Model file for the job. Use its own axes, mm. A direction names the side the tool comes from. Give positions to 0.01 mm unless a question says otherwise; leave off trailing zeros. Write each loop counter-clockwise with the first axis right and the second up, starting at its lowest first coordinate (ties: lowest second). Pieces come first, ordered by that corner, then holes. Notation, with made-up numbers: (19.25, -13.5) - (37.25, -13.5) arc R34 cw to (37.25, 21.5) - close; hole circle Ø2 at (37, 56). An arc over 180 degrees is marked (long way). Use a Markdown table: item, result. Add a question column.
```python
from build123d import *

# Parameters (mm, degrees)
F1_R   = 4.7553681228
F1_R_2 = 2.331332345


with BuildPart() as f2:
    # F2: sweep along a path in F0
    with BuildLine(Plane.XY) as f2_path:
        Line((0, 0), (0, 11.7783713439))
        ThreePointArc((0, 11.7783713439), (0.4385311413, 13.8260534118), (1.6772007405, 15.514546538))
        Line((1.6772007405, 15.514546538), (17.2961814494, 29.405420182))
        ThreePointArc((17.2961814494, 29.405420182), (18.5348510486, 31.0939133082), (18.9733821899, 33.1415953761))
        Line((18.9733821899, 33.1415953761), (18.9733821899, 52.8334341943))
    # F1 (on Front) → F2 (sweep)
    with BuildSketch(Plane.XZ):
        Circle(F1_R)
        Circle(F1_R_2, mode=Mode.SUBTRACT)
    sweep(path=f2_path.line)

    # F3 (on Right) → F4 (revolve)
    with BuildSketch(Plane.YZ):
        with BuildLine():
            Line((-4.0508554065, -8), (-4.0508554065, 0))
            Line((-4.0508554065, 0), (-4.0508554065, 8))
            ThreePointArc((-4.0508554065, 8), (-12.0508554065, 0), (-4.0508554065, -8))
        make_face()
    revolve(axis=Axis((0, -4.0508554065, 4), (0, 0, 1)))


solid = f2.part
```
(1) Band-saw the part on A-A (z = 0). Write the cut outline in (x, y).
(2) Two-plate mould, pull along X, no slides. Class faces 3 (the flat face through (21.2, 52.833, 1.1)), 4 (the cylindrical face through (17.94, 43.13, 4.64)), 5 (the cylindrical face through (-1.85, 7.75, 1.42)): +X half, -X half, draft (parallel to the pull), parting line (faces both ways), or undercut.
(3) Which spindle directions (+Z, -Z, +X, -X, +Y, -Y) get a long thin tool onto all of the face, cutting with end or side? Do faces 1 (the cylindrical face through (21.197, 43.125, -0.7)), 2 (the cylindrical face through (-1.031, 7.146, 4.642)). Say none if no direction does.
(4) Band-saw the part on C-C (z = -3). Write the cut outline in (x, y).
(5) Flat gauge pins, fed straight in: pin 1 (8 mm diameter, centred on x = 19.5, z = 4, fed in from -Y); pin 2 (3 mm diameter, centred on y = 2.5, z = -0.5, fed in from +X); pin 3 (3.5 mm diameter, centred on x = 18.97, z = 0, fed in from +Y). Where does each tip first touch, or does it go through?
(6) Probe probe 1 along Z at (x, y) = (0, 9.5); probe 2 along X at (y, z) = (44.25, 0). List the from-to ranges inside material, lowest first. Write a range as [from, to].
(7) Band-saw the part on D-D (x = 6). Give the number of separate pieces and of enclosed holes in the cut face, then the cut area to 3 significant figures.
(8) Band-saw the part on B-B (y = 1). Write the cut outline in (x, z).
Model answer:
| question | item | result |
|---|---|---|
| 1 | outline | (-4.76, 2.38) arc R8 ccw (long way) to (4.76, 2.38) - (4.76, 11.78) arc R0.24 cw to (4.84, 11.96) - (20.46, 25.85) arc R9.76 ccw to (23.73, 33.14) - (23.73, 52.83) - (21.3, 52.83) - (21.3, 33.14) arc R7.33 cw to (18.85, 27.66) - (3.23, 13.77) arc R2.67 ccw to (2.33, 11.78) - (2.33, 3.6) arc R8 ccw to (-2.33, 3.6) - (-2.33, 11.78) arc R7.33 cw to (0.13, 17.26) - (15.75, 31.15) arc R2.67 ccw to (16.64, 33.14) - (16.64, 52.83) - (14.22, 52.83) - (14.22, 33.14) arc R0.24 cw to (14.14, 32.96) - (-1.48, 19.07) arc R9.76 ccw to (-4.76, 11.78) - close |
| 2 | face 3 | draft |
| 2 | face 4 | parting line |
| 2 | face 5 | undercut |
| 3 | face 1 | +Y |
| 3 | face 2 | none |
| 4 | outline | (-3.69, 2.38) arc R7.42 ccw (long way) to (3.69, 2.38) - (3.69, 11.78) arc R1.31 cw to (4.13, 12.76) - (19.75, 26.65) arc R8.69 ccw to (22.66, 33.14) - (22.66, 52.83) - (15.28, 52.83) - (15.28, 33.14) arc R1.31 cw to (14.84, 32.16) - (-0.77, 18.27) arc R8.69 ccw to (-3.69, 11.78) - close |
| 5 | pin 1 | stops at y = 22.5 |
| 5 | pin 2 | stops at x = 6.19 |
| 5 | pin 3 | stops at y = 30.27 |
| 6 | probe 1 | z = [-4.76, -2.33], [2.33, 4.76] |
| 6 | probe 2 | x = [14.22, 16.64], [21.3, 23.73] |
| 7 | separate pieces | 2 |
| 7 | enclosed holes | 1 |
| 7 | area | 160 mm^2 |
| 8 | outline | circle Ø12.41 at (0, 0) |
